from build123d import *

# Parameters (mm, degrees)
BOSS_EXTRUDE1_DEPTH      = 9.6774
BOSS_EXTRUDE1_DEPTH_BACK = 9.6774
SKETCH2_R                = 6.4516
BOSS_EXTRUDE2_DEPTH      = 4.8387
SKETCH3_R                = 4.8387
CUT_EXTRUDE1_DEPTH       = 30.0322
FILLET1_R                = 0.80772
SKETCH4_R                = 1.6129
CUT_EXTRUDE2_DEPTH       = 1.20904


with BuildPart() as part:
    # Sketch1 → Boss-Extrude1 (new body, two sides)
    with BuildSketch(Plane(origin=(0, 0, 0), x_dir=(0, 0, -1), z_dir=(1, 0, 0))) as boss_extrude1_sk:
        with BuildLine():
            Line((-7.25932, 3.512610623), (-7.25932, -3.512610623))
            ThreePointArc((-7.25932, -3.512610623), (0, -8.0645), (7.25932, -3.512610623))
            Line((7.25932, -3.512610623), (7.25932, 3.512610623))
            ThreePointArc((7.25932, 3.512610623), (0, 8.0645), (-7.25932, 3.512610623))
        make_face()
    extrude(amount=BOSS_EXTRUDE1_DEPTH)
    extrude(boss_extrude1_sk.sketch, amount=-BOSS_EXTRUDE1_DEPTH_BACK)

    # Sketch2 → Boss-Extrude2 (add)
    with BuildSketch(Plane(origin=(9.6774, 0, 0), x_dir=(0, 0, -1), z_dir=(1, 0, 0))):
        Circle(SKETCH2_R)
    boss_extrude2 = extrude(amount=BOSS_EXTRUDE2_DEPTH)

    # Mirror1: Boss-Extrude2 across plane
    add(boss_extrude2.mirror(Plane(origin=(0, 0, 0), x_dir=(0, 0, 1), z_dir=(1, 0, 0))))

    # Sketch3 → Cut-Extrude1 (cut, through all)
    with BuildSketch(Plane(origin=(14.5161, 0, 0), x_dir=(0, 0, -1), z_dir=(1, 0, 0))):
        Circle(SKETCH3_R)
    extrude(amount=-CUT_EXTRUDE1_DEPTH, mode=Mode.SUBTRACT)

    # Fillet1
    fillet1_edges = [part.edges().sort_by_distance(p)[0] for p in [
        (14.5161, 0, 6.4516),
        (-14.5161, 0, 6.4516),
    ]]
    fillet(fillet1_edges, radius=FILLET1_R)

    # Sketch4 → Cut-Extrude2 (cut)
    with BuildSketch(Plane.XY.offset(7.25932)):
        Circle(SKETCH4_R)
    extrude(amount=-CUT_EXTRUDE2_DEPTH, mode=Mode.SUBTRACT)


solid = part.part
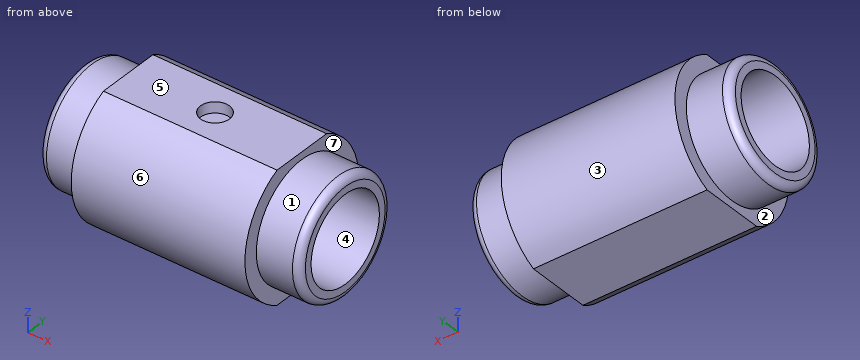
Here's how the part is built. I have some questions about the finished solid (model axes, mm). Face numbers are marked on the shaded views. A direction names the side the tool comes from. Round coordinates to 2 decimals unless told otherwise and drop trailing zeros. Loops run counter-clockwise (first coordinate to the right, second up) from the corner with the lowest first, then second, coordinate; pieces in that order, holes last. Notation, with made-up numbers: (-6.75, 49.25) - (-0.75, 49.25) arc R10 cw to (-0.75, 68.25) - close; hole circle Ø9 at (-10, 5). An arc over 180 degrees is marked (long way). One line per question, with ' | ' between items. Start each with the question number.
Q1. Will these pins go through, and if not, where does the flat tip stop? pin 1 (5 mm diameter, centred on x = -10, z = 5, fed in from -Y); pin 2 (3 mm diameter, centred on x = -9, y = 6, fed in from +Z); pin 3 (1.5 mm diameter, centred on x = 4.5, z = 3, fed in from +Y); pin 4 (1.5 mm diameter, centred on y = -3.5, z = -3, fed in from -X).
Q2. I want a section at B-B (x = 0). Write out the boundary of the cut face in (y, z).
Q3. I want a section at A-A (z = 0). Write out the boundary of the cut face in (x, y), then the cut area to 3 significant figures.
Q4. We'd pull the mould along Z, two halves only. Please class the marked faces 4, 5, 6 and 7: +Z half, -Z half, draft (parallel to the pull), parting line (faces both ways), or undercut.
Q5. I want a section at C-C (y = 0). Write out the boundary of the cut face in (x, z), then the cut area to 3 significant figures.
Q6. Please list where these lines run through material, in increasing order: line 1 (Y direction, x = -9.75, z = 0.25); line 2 (Y direction, x = -7.75, z = 0); line 3 (Z direction, x = -2, y = 4). Write a range as [from, to].
Q7. For the marked faces 1, 2 and 3, which set-ups out of +Z, -Z, +X, -X, +Y, -Y let a thin tool reach every point of the face, with its end or its side?
Q8. I want a section at D-D (x = 3.25). Write out the boundary of the cut face in (y, z).
Response values:
1) pin 1: stops at y = -7.66 | pin 2: stops at z = 6.69 | pin 3: stops at y = 7.74 | pin 4: stops at x = -14.52
2) outline: (-3.51, -7.26) - (3.51, -7.26) arc R8.06 ccw to (3.51, 7.26) - (1.61, 7.26) - (1.61, 6.05) - (-1.61, 6.05) - (-1.61, 7.26) - (-3.51, 7.26) arc R8.06 ccw to start; hole circle Ø9.68 at (0, 0)
3) outline: (-14.52, -5.64) arc R0.81 ccw to (-13.71, -6.45) - (-9.68, -6.45) - (-9.68, -8.06) - (9.68, -8.06) - (9.68, -6.45) - (13.71, -6.45) arc R0.81 ccw to (14.52, -5.64) - (14.52, -4.84) - (-14.52, -4.84) - close; (-14.52, 4.84) - (14.52, 4.84) - (14.52, 5.64) arc R0.81 ccw to (13.71, 6.45) - (9.68, 6.45) - (9.68, 8.06) - (-9.68, 8.06) - (-9.68, 6.45) - (-13.71, 6.45) arc R0.81 ccw to (-14.52, 5.64) - close | area: 156 mm²
4) face 4: undercut | face 5: +Z half | face 6: parting line | face 7: draft
5) outline: (-14.52, -5.64) arc R0.81 ccw to (-13.71, -6.45) - (-9.68, -6.45) - (-9.68, -7.26) - (9.68, -7.26) - (9.68, -6.45) - (13.71, -6.45) arc R0.81 ccw to (14.52, -5.64) - (14.52, -4.84) - (-14.52, -4.84) - close; (-14.52, 4.84) - (14.52, 4.84) - (14.52, 5.64) arc R0.81 ccw to (13.71, 6.45) - (9.68, 6.45) - (9.68, 7.26) - (1.61, 7.26) - (1.61, 6.05) - (-1.61, 6.05) - (-1.61, 7.26) - (-9.68, 7.26) - (-9.68, 6.45) - (-13.71, 6.45) arc R0.81 ccw to (-14.52, 5.64) - close | area: 120 mm²
6) line 1: y = [-6.45, -4.83], [4.83, 6.45] | line 2: y = [-8.06, -4.84], [4.84, 8.06] | line 3: z = [-7, -2.72], [2.72, 7]
7) face 1: +X | face 2: -X | face 3: +X, -X, +Y
8) outline: (-3.51, -7.26) - (3.51, -7.26) arc R8.06 ccw to (3.51, 7.26) - (-3.51, 7.26) arc R8.06 ccw to start; hole circle Ø9.68 at (0, 0)
